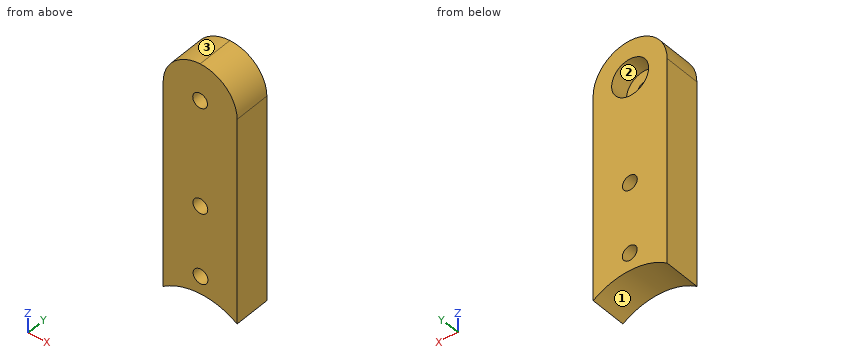
from build123d import *

# Parameters (mm, degrees)
SKETCH_1_W          = 4
SKETCH_1_H          = 15
EXTRUDE_1_DEPTH     = 2
SKETCH_3_R          = 0.4
CUT_EXTRUDE_1_DEPTH = 16.652475842
SKETCH_3_3_R        = 1
CUT_EXTRUDE_2_DEPTH = 1
SKETCH_4_R          = 3.5
CUT_EXTRUDE_3_DEPTH = 16.652475842
FILLET_1_R          = 2


with BuildPart() as part:
    # 草图1 → 凸台-拉伸1 (new body)
    with BuildSketch(Plane(origin=(0, 0, 0), x_dir=(1, 0, 0), z_dir=(0, 1, 0))):
        with Locations((2, -7.5)):
            Rectangle(SKETCH_1_W, SKETCH_1_H)
    extrude(amount=EXTRUDE_1_DEPTH)

    # 草图3 → 切除-拉伸1 (cut, through all)
    with BuildSketch(Plane(origin=(0, 2, 0), x_dir=(1, 0, 0), z_dir=(0, 1, 0))):
        with Locations(Location((2, -13, 0), (0, 0, 270))):
            Circle(SKETCH_3_R)
        with Locations(Location((2.022495613, -3.450026495, 0), (0, 0, 270))):
            Circle(SKETCH_3_R)
        with Locations(Location((2.013497368, -7.270015897, 0), (0, 0, 270))):
            Circle(SKETCH_3_R)
    extrude(amount=-CUT_EXTRUDE_1_DEPTH, mode=Mode.SUBTRACT)

    # 草图3<3> → 切除-拉伸2 (cut)
    with BuildSketch(Plane(origin=(0, 2, 0), x_dir=(1, 0, 0), z_dir=(0, 1, 0))):
        with Locations(Location((2, -13, 0), (0, 0, 270))):
            Circle(SKETCH_3_3_R)
    extrude(amount=-CUT_EXTRUDE_2_DEPTH, mode=Mode.SUBTRACT)

    # 草图4 → 切除-拉伸3 (cut, through all)
    with BuildSketch(Plane(origin=(0, 2, 0), x_dir=(1, 0, 0), z_dir=(0, 1, 0))):
        with Locations((2, 1)):
            Circle(SKETCH_4_R)
    extrude(amount=-CUT_EXTRUDE_3_DEPTH, mode=Mode.SUBTRACT)

    # 圆角1
    fillet_1_edges = [part.edges().sort_by_distance(p)[0] for p in [
        (4, 1, 15),
        (0, 1, 15),
    ]]
    fillet(fillet_1_edges, radius=FILLET_1_R - 0.0001)  # a hair under: the kernel refuses the full size


solid = part.part
For this review, take the finished solid that the model builds, in its own axes (mm). Face numbers are marked on the shaded views. Round coordinates to 2 decimals unless told otherwise and drop trailing zeros. Loops run counter-clockwise (first coordinate to the right, second up) from the corner with the lowest first, then second, coordinate; pieces in that order, holes last. Notation, with made-up numbers: (70, 52.5) - (99, 52.5) arc R17 ccw to (99, 76.5) - close; hole circle Ø4 at (-32.5, 45). An arc over 180 degrees is marked (long way). Put each result on its own line as item: value. Start each with the question number.
1. Mouldability with a two-part tool opening along Z and no side actions: class the marked faces 1, 2 and 3 as +Z half, -Z half, draft (parallel to the pull), parting line (faces both ways), or undercut.
2. Consider section B-B on z = 3.5. State the section outline as (x, y) points, plus the area to 3 significant figures.
3. For probe 1 along X at (y, z) = (1.3, 13); probe 2 along X at (y, z) = (0.4, 13); probe 3 along Z at (x, y) = (1.4, 1.85), list the stretches that pass through material, from the lowest coordinate up. Write a range as [from, to].
4. Consider section A-A on x = 1.75. State the section outline as (y, z) points, plus the area to 3 significant figures.
5. Insertion check: P1, Ø1.8, axis at x = 2, z = 13, coming from the +Y side. The pin has a flat end and moves straight along its axis. Give the tip position at first contact, or say it passes through.
6. Consider section C-C on x = 2.65. State the section outline as (y, z) points.
7. Consider section D-D on y = 0.4. State how many separate pieces and enclosed holes the cut face has, plus the area to 3 significant figures.
Result sheet:
1. face 1: -Z half
1. face 2: undercut
1. face 3: +Z half
2. outline: (0, 0) - (1.63, 0) - (1.63, 2) - (0, 2) - close; (2.42, 0) - (4, 0) - (4, 2) - (2.42, 2) - close
2. area: 6.41 mm^2
3. probe 1: [0, 1], [3, 4]
3. probe 2: [0, 1.6], [2.4, 4]
3. probe 3: [2.45, 12.2], [13.8, 14.91]
4. outline: (0, 2.49) - (2, 2.49) - (2, 3.16) - (0, 3.16) - close; (0, 3.74) - (2, 3.74) - (2, 6.97) - (0, 6.97) - close; (0, 7.57) - (2, 7.57) - (2, 12.03) - (1, 12.03) - (1, 12.69) - (0, 12.69) - close; (0, 13.31) - (1, 13.31) - (1, 13.97) - (2, 13.97) - (2, 14.98) - (0, 14.98) - close
4. area: 20.1 mm^2
5. P1: y = 1
6. outline: (0, 2.44) - (2, 2.44) - (2, 12.24) - (1, 12.24) - (1, 13.76) - (2, 13.76) - (2, 14.89) - (0, 14.89) - close
7. separate pieces: 1
7. enclosed holes: 3
7. area: 47.6 mm^2
